```python
from build123d import *

# Parameters (mm, degrees)
SKETCH_W           = 40
SKETCH_H           = 40
PAD_DEPTH          = 50
POCKET_DEPTH       = 150.997689
POCKET_DEPTH_BACK  = 200.997689
POLARPATTERN_COUNT = 4


with BuildPart() as part:
    # Sketch → Pad (new body)
    with BuildSketch(Plane.XY):
        Rectangle(SKETCH_W, SKETCH_H)
    extrude(amount=PAD_DEPTH)

    # Sketch001 → Pocket (cut, two sides)
    with BuildSketch(Plane.XY) as pocket_sk:
        Polygon((-19.717157, 20), (-16.717157, 17), (-12.6, 17), (-12.6, 16.6), (-16.6, 16.6), (-16.6, 12.6), (-17, 12.6), (-17, 16.717157), (-20, 19.717157), (-20, 20), align=None)
    pocket = extrude(amount=-POCKET_DEPTH, mode=Mode.SUBTRACT) + extrude(pocket_sk.sketch, amount=POCKET_DEPTH_BACK, mode=Mode.SUBTRACT)

    # PolarPattern: Pocket ×4 about axis
    polarpattern_axis = Axis((0, 0, 0), (0, 0, 1))
    for i in range(1, POLARPATTERN_COUNT):
        add(pocket.rotate(polarpattern_axis, i * 360 / POLARPATTERN_COUNT), mode=Mode.SUBTRACT)


solid = part.part
```
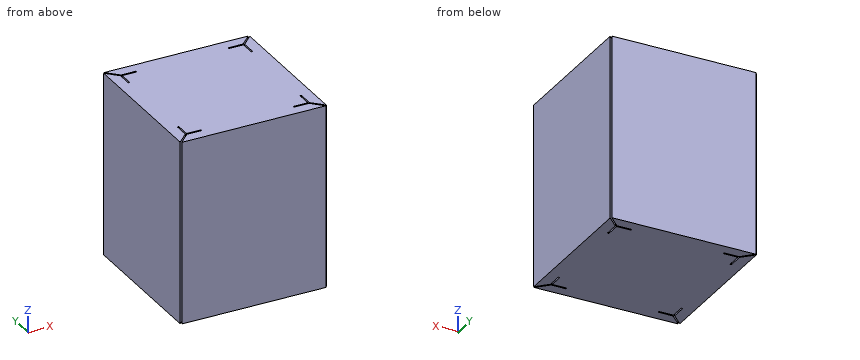
Work out the finished part from the listing and answer in its coordinate system (mm). Give positions to 0.01 mm unless a question says otherwise; leave off trailing zeros. Order: outer loops, then holes, each group sorted by start corner. A loop starts at its lowest first (then second) coordinate and runs counter-clockwise, first axis right, second up.
1. Section A-A, the plane x = -15.5 is taken. Determine the outline of the cut face in (y, z).
Result sheet:
outline: (-20, 0) - (-17, 0) - (-17, 50) - (-20, 50) - close; (-16.6, 0) - (16.6, 0) - (16.6, 50) - (-16.6, 50) - close; (17, 0) - (20, 0) - (20, 50) - (17, 50) - close
2. This flat-tipped pin is pushed along its axis until it touches: P1, Ø8, axis at x = -11.5, y = 0.5, coming from the -Z side. Where does it stop, or does it pass through?
Result sheet:
P1: stops at z = 0
3. A straight line is drawn through the part: L1, parallel to Y at x = -13, z = 26. Find the intervals that lie inside material, in ascending order.
Result sheet:
L1: y = -20 to -17, -16.6 to 16.6, 17 to 20
